Could you check a few things on this model? Use its own coordinates, in mm. Face numbers are marked on the shaded views. A direction names the side the tool comes from. Round coordinates to 2 decimals unless told otherwise and drop trailing zeros. Loops run counter-clockwise (first coordinate to the right, second up) from the corner with the lowest first, then second, coordinate; pieces in that order, holes last. Notation, with made-up numbers: (-12.75, -32.75) - (15.25, -32.75) arc R9 cw to (15.25, -21.75) - close; hole circle Ø9 at (38.25, -18.75). An arc over 180 degrees is marked (long way). Answer as CSV lines item,"result". Start each with the question number.
1) Suppose I cut it at A-A, the plane x = 10. Write out the boundary of the cut face in (y, z), then the cut area to 3 significant figures.
2) I'm going to push flat-ended pins straight in: pin 1 Ø8 at (x, y) = (8, -12) entering from +Z; pin 2 Ø6 at (x, z) = (9.5, 13.5) entering from -Y (3 decimals); pin 3 Ø8 at (x, z) = (8.5, 12.5) entering from +Y. Where does each tip first touch, or does it pass through?
3) Which directions (+Z, -Z, +X, -X, +Y, -Y) give clear straight access to the entire face, cutting with the end or side of a thin tool? Please do the marked faces 4 and 5.
4) Suppose I cut it at D-D, the plane x = 2.5. Write out the boundary of the cut face in (y, z), then the cut area to 3 significant figures.
5) Suppose I cut it at C-C, the plane z = 4. Count the separate pieces of the cut face and the enclosed holes in it, then the cut area to 3 significant figures.
6) We'd pull the mould along Y, two halves only. Please class the marked faces 1, 2 and 3: pulls with the +Y half, pulls with the -Y half, needs draft (parallel to the pull), parting line crosses it, or undercut.
7) Please list where these lines run through material, in increasing order: line 1 along Y through (x, z) = (10, 2.8); line 2 along Z through (x, y) = (17.5, 42.5); line 3 along Y through (x, z) = (2.5, 5.5).
8) Suppose I cut it at B-B, the plane y = 0. Write out the boundary of the cut face in (x, z).
```python
from build123d import *

# Parameters (mm, degrees)
REVOLVE1_ANGLE      = 180
BOSS_EXTRUDE3_DEPTH = 5
BOSS_EXTRUDE4_DEPTH = 5
SKETCH17_R          = 2.2479
CUT_EXTRUDE1_DEPTH  = 34
CHAMFER1_SIZE       = 0.5


with BuildPart() as part:
    # Sketch1 → Revolve1 (revolve)
    with BuildSketch(Plane.XY):
        Polygon((15, 26), (15, 26.75), (18, 25), (20, 25), (20, 33), (0, 33), (0, 26), align=None)
    revolve(axis=Axis((0, 0, 0), (1, 0, 0)), revolution_arc=REVOLVE1_ANGLE)

    # Sketch9 → Boss-Extrude3 (add)
    with BuildSketch(Plane(origin=(0, 0, 0), x_dir=(-1, 0, 0), z_dir=(0, 0, -1))):
        with BuildLine():
            Line((-20, 29), (0, 29))
            Line((0, 29), (0, 38))
            ThreePointArc((0, 38), (-10, 48), (-20, 38))
            Line((-20, 38), (-20, 29))
        make_face()
    extrude(amount=-BOSS_EXTRUDE3_DEPTH)

    # Sketch11 → Boss-Extrude4 (add)
    with BuildSketch(Plane(origin=(0, 0, 0), x_dir=(-1, 0, 0), z_dir=(0, 0, -1))):
        with BuildLine():
            Line((-20, -29), (0, -29))
            Line((0, -29), (0, -38))
            ThreePointArc((0, -38), (-10, -48), (-20, -38))
            Line((-20, -38), (-20, -29))
        make_face()
    extrude(amount=-BOSS_EXTRUDE4_DEPTH)

    # Sketch17 → Cut-Extrude1 (cut, through all)
    with BuildSketch(Plane(origin=(0, 0, 0), x_dir=(-1, 0, 0), z_dir=(0, 0, -1))):
        with Locations((-10, 38)):
            Circle(SKETCH17_R)
        with Locations((-10, -38)):
            Circle(SKETCH17_R)
    extrude(amount=-CUT_EXTRUDE1_DEPTH, mode=Mode.SUBTRACT)

    # Chamfer1
    chamfer1_edges = [part.edges().sort_by_distance(p)[0] for p in [
        (20, 0, 25),
    ]]
    chamfer(chamfer1_edges, length=CHAMFER1_SIZE)


solid = part.part
```
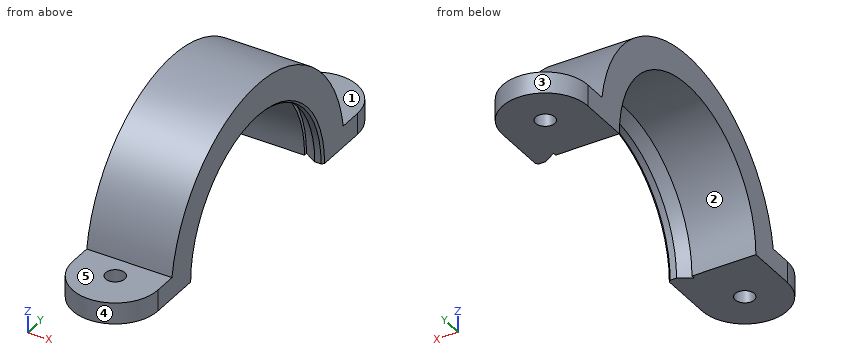
Filled sheet:
1,outline,"(-48, 0) - (-40.25, 0) - (-40.25, 5) - (-48, 5) - close; (-35.75, 0) - (-26, 0) arc R26 cw to (26, 0) - (35.75, 0) - (35.75, 5) - (32.62, 5) arc R33 ccw to (-32.62, 5) - (-35.75, 5) - close; (40.25, 0) - (48, 0) - (48, 5) - (40.25, 5) - close"
1,area,"755 mm²"
2,pin 1,"z = 32.02"
2,pin 2,"y = -31.285"
2,pin 3,"y = 31.89"
3,face 4,"+Z, -Z, -Y"
3,face 5,"+Z, +X, -X, -Y"
4,outline,"(-44.61, 0) - (-26, 0) arc R26 cw to (26, 0) - (44.61, 0) - (44.61, 5) - (32.62, 5) arc R33 ccw to (-32.62, 5) - (-44.61, 5) - close"
4,area,"766 mm²"
5,separate pieces,"2"
5,enclosed holes,"2"
5,area,"779 mm²"
6,face 1,"needs draft"
6,face 2,"undercut"
6,face 3,"pulls with the +Y half"
7,line 1,"-48 to -40.25, -35.75 to -25.85, 25.85 to 35.75, 40.25 to 48"
7,line 2,"0 to 5"
7,line 3,"-32.54 to -25.41, 25.41 to 32.54"
8,outline,"(0, 26) - (15, 26) - (15, 26.75) - (18, 25) - (19.5, 25) - (20, 25.5) - (20, 33) - (0, 33) - close"
